from build123d import *

# Parameters (mm, degrees)
SKETCH1_W               = 125
SKETCH1_H               = 55
SKETCH1_R               = 3.25
BOSS_EXTRUDE1_DEPTH     = 8
SKETCH5_R               = 5.5
CUT_EXTRUDE1_DEPTH      = 6
SKETCH3_W               = 55
SKETCH3_H               = 8
BOSS_EXTRUDE3_DEPTH     = 10
SKETCH4_W               = 5
SKETCH4_H               = 55
BOSS_EXTRUDE4_DEPTH     = 50
CUT_EXTRUDE2_DEPTH      = 150.483276657
CUT_EXTRUDE2_DEPTH_BACK = 150.483276657
SKETCH6_R               = 6
SKETCH6_R_2             = 2.5
SKETCH8_R               = 1.5
CUT_EXTRUDE3_DEPTH      = 10


with BuildPart() as part:
    # Sketch1 → Boss-Extrude1 (new body)
    with BuildSketch(Plane(origin=(0, 0, 0), x_dir=(1, 0, 0), z_dir=(0, 1, 0))):
        Rectangle(SKETCH1_W, SKETCH1_H)
        with Locations(Location((-52.5, 17.5, 0), (0, 0, 270))):
            Circle(SKETCH1_R, mode=Mode.SUBTRACT)
        with Locations(Location((-52.5, -17.5, 0), (0, 0, 90))):
            Circle(SKETCH1_R, mode=Mode.SUBTRACT)
        with Locations(Location((-17.5, -17.5, 0), (0, 0, 270))):
            Circle(SKETCH1_R, mode=Mode.SUBTRACT)
        with Locations(Location((-17.5, 17.5, 0), (0, 0, 90))):
            Circle(SKETCH1_R, mode=Mode.SUBTRACT)
        with Locations(Location((52.5, -17.5, 0), (0, 0, 270))):
            Circle(SKETCH1_R, mode=Mode.SUBTRACT)
        with Locations(Location((17.5, -17.5, 0), (0, 0, 90))):
            Circle(SKETCH1_R, mode=Mode.SUBTRACT)
        with Locations(Location((17.5, 17.5, 0), (0, 0, 270))):
            Circle(SKETCH1_R, mode=Mode.SUBTRACT)
        with Locations(Location((52.5, 17.5, 0), (0, 0, 90))):
            Circle(SKETCH1_R, mode=Mode.SUBTRACT)
    extrude(amount=BOSS_EXTRUDE1_DEPTH)

    # Sketch5 → Cut-Extrude1 (cut)
    with BuildSketch(Plane(origin=(0, 8, 0), x_dir=(1, 0, 0), z_dir=(0, 1, 0))):
        with Locations(Location((-52.5, 17.5, 0), (0, 0, 270))):
            Circle(SKETCH5_R)
        with Locations(Location((-17.5, 17.5, 0), (0, 0, 270))):
            Circle(SKETCH5_R)
        with Locations(Location((17.5, 17.5, 0), (0, 0, 270))):
            Circle(SKETCH5_R)
        with Locations(Location((52.5, 17.5, 0), (0, 0, 270))):
            Circle(SKETCH5_R)
        with Locations(Location((52.5, -17.5, 0), (0, 0, 270))):
            Circle(SKETCH5_R)
        with Locations(Location((17.5, -17.5, 0), (0, 0, 270))):
            Circle(SKETCH5_R)
        with Locations(Location((-17.5, -17.5, 0), (0, 0, 270))):
            Circle(SKETCH5_R)
        with Locations(Location((-52.5, -17.5, 0), (0, 0, 270))):
            Circle(SKETCH5_R)
    extrude(amount=-CUT_EXTRUDE1_DEPTH, mode=Mode.SUBTRACT)

    # Sketch3 → Boss-Extrude3 (add)
    with BuildSketch(Plane.ZY.offset(62.5)):
        with Locations((0, 4)):
            Rectangle(SKETCH3_W, SKETCH3_H)
    extrude(amount=BOSS_EXTRUDE3_DEPTH)

    # Sketch4 → Boss-Extrude4 (add)
    with BuildSketch(Plane(origin=(0, 8, 0), x_dir=(1, 0, 0), z_dir=(0, 1, 0))):
        with Locations((-70, 0)):
            Rectangle(SKETCH4_W, SKETCH4_H)
        with Locations((37.5, 0)):
            Rectangle(SKETCH4_W, SKETCH4_H)
    extrude(amount=BOSS_EXTRUDE4_DEPTH)

    # Sketch6 → Cut-Extrude2 (cut, two sides: drawn at the far end of the back side and taken through both)
    with BuildSketch(Plane.ZY.offset(72.5).offset(-CUT_EXTRUDE2_DEPTH_BACK)):
        with Locations((0, 33)):
            Circle(SKETCH6_R)
        with Locations((-18.5, 33)):
            Circle(SKETCH6_R_2)
        with Locations((18.5, 33)):
            Circle(SKETCH6_R_2)
    extrude(amount=CUT_EXTRUDE2_DEPTH + CUT_EXTRUDE2_DEPTH_BACK, mode=Mode.SUBTRACT)

    # Sketch8 → Cut-Extrude3 (cut)
    with BuildSketch(Plane(origin=(40, 0, 0), x_dir=(0, 0, -1), z_dir=(1, 0, 0))):
        with Locations((9.525, 33)):
            Circle(SKETCH8_R)
        with Locations((-9.525, 33)):
            Circle(SKETCH8_R)
    extrude(amount=-CUT_EXTRUDE3_DEPTH, mode=Mode.SUBTRACT)


solid = part.part
Build history of the part. All positions in model axes, mm. A direction names the side the tool comes from. Round coordinates to 2 decimals unless told otherwise and drop trailing zeros. Write each loop counter-clockwise with the first axis right and the second up, starting at its lowest first coordinate (ties: lowest second). Pieces come first, ordered by that corner, then holes. Notation, with made-up numbers: (52, -30) - (99, -30) arc R24 cw to (99, -7) - close; hole circle Ø7 at (17.5, 50.25). An arc over 180 degrees is marked (long way). One line per question, with ' | ' between items.
1. Band-saw the part on D-D, the plane y = 37. Write the cut outline in (x, z).
Results are:
outline: (-72.5, -27.5) - (-67.5, -27.5) - (-67.5, -4.47) - (-72.5, -4.47) - close; (-72.5, 4.47) - (-67.5, 4.47) - (-67.5, 27.5) - (-72.5, 27.5) - close; (35, -27.5) - (40, -27.5) - (40, -4.47) - (35, -4.47) - close; (35, 4.47) - (40, 4.47) - (40, 27.5) - (35, 27.5) - close
2. Band-saw the part on C-C, the plane x = -17.5. Write the cut outline in (y, z), and give its area (3 significant figures).
Results are:
outline: (0, -27.5) - (8, -27.5) - (8, -23) - (2, -23) - (2, -20.75) - (0, -20.75) - close; (0, -14.25) - (2, -14.25) - (2, -12) - (8, -12) - (8, 12) - (2, 12) - (2, 14.25) - (0, 14.25) - close; (0, 20.75) - (2, 20.75) - (2, 23) - (8, 23) - (8, 27.5) - (0, 27.5) - close | area: 282 mm^2
3. Drop flat-ended pins along their axis: pin 1 Ø5 at (x, z) = (27, -2) entering from +Y; pin 2 Ø10 at (x, z) = (17.5, -17.5) entering from +Y; pin 3 Ø10 at (y, z) = (41, 1) entering from +X. Give the stop position or say it passes through.
Results are:
pin 1: y = 8 | pin 2: y = 2 | pin 3: x = 40
4. Drill centre lines: line 1 along X through (y, z) = (1.25, 17.5); line 2 along Z through (x, y) = (17.5, 1.4); line 3 along Y through (x, z) = (39, 18.5). Where is each one in solid material? Low to high. Write a range as from..to.
Results are:
line 1: -72.5..-55.75, -49.25..-20.75, -14.25..14.25, 20.75..49.25, 55.75..62.5 | line 2: -27.5..-20.75, -14.25..14.25, 20.75..27.5 | line 3: 0..30.5, 35.5..58
5. Mould opens along X. For faces 4 (the face through (-4, 0, 0)), 5 (the face through (-20, 2, 20)) say: released by +X, released by -X, zero draft, split by the parting line, or undercut.
Results are:
face 4: zero draft | face 5: undercut
6. Band-saw the part on B-B, the plane y = 19.5. Write the cut outline in (x, z), and give its area (3 significant figures).
Results are:
outline: (-72.5, -27.5) - (-67.5, -27.5) - (-67.5, 27.5) - (-72.5, 27.5) - close; (35, -27.5) - (40, -27.5) - (40, 27.5) - (35, 27.5) - close | area: 550 mm^2
7. Tool access for faces 1 (the face through (-70, 58, 0)), 2 (the face through (15, 2, -15)), 3 (the face through (35, 32.6, 6.5)): list every direction of +Z, -Z, +X, -X, +Y, -Y with a clear straight run to the whole face (end or side of a thin tool).
Results are:
face 1: +Z, -Z, +X, -X, +Y | face 2: +Y | face 3: +Z, -Z, +Y
8. Band-saw the part on A-A, the plane z = 0. Write the cut outline in (x, y).
Results are:
outline: (-72.5, 0) - (62.5, 0) - (62.5, 8) - (40, 8) - (40, 27) - (35, 27) - (35, 8) - (-67.5, 8) - (-67.5, 27) - (-72.5, 27) - close; (-72.5, 39) - (-67.5, 39) - (-67.5, 58) - (-72.5, 58) - close; (35, 39) - (40, 39) - (40, 58) - (35, 58) - close
